Source: CAD feature listing. Evaluate the final solid. Frame: model axes, mm. Give positions to 0.01 mm unless a question says otherwise; leave off trailing zeros. Write each loop counter-clockwise with the first axis right and the second up, starting at its lowest first coordinate (ties: lowest second). Pieces come first, ordered by that corner, then holes. Notation, with made-up numbers: M 40.5,36.5 L 93.5,36.5 A38 ccw 93.5,75.5 Z; hole C 67.25,55.5 d6. An arc over 180 degrees is marked long. Use CSV: the item, a comma, the result in double quotes. Start each with the question number.
from build123d import *

# Parameters (mm, degrees)
F0_R     = 3.302961
F1_DEPTH = 3.81
F2_R     = 2.241818
F3_DEPTH = 12.7
F4_R     = 3.347199
F5_DEPTH = 3.81


with BuildPart() as f1:
    # F0 (on Front) → F1 (new body)
    with BuildSketch(Plane.XZ):
        Circle(F0_R)
    extrude(amount=-F1_DEPTH)

    # F2 (on face) → F3 (join)
    with BuildSketch(Plane(origin=(0, 3.81, 0), x_dir=(-1, 0, 0), z_dir=(0, 1, 0))):
        Circle(F2_R)
    extrude(amount=F3_DEPTH)

    # F4 (on face) → F5 (join)
    with BuildSketch(Plane(origin=(0, 16.51, 0), x_dir=(-1, 0, 0), z_dir=(0, 1, 0))):
        Circle(F4_R)
    extrude(amount=F5_DEPTH)


solid = f1.part
1. Section A-A on z = 3. Return loops of the section in (x, y), then the cut area to 3 significant figures.
2. First-contact query: pin 1 (4 mm diameter, centred on y = 13.5, z = 0.5, fed in from -X). Flat tip, straight axial feed; report the tip coordinate or a pass-through.
3. Section D-D on y = 13.75. Return loops of the section in (x, z), then the cut area to 3 significant figures.
4. Section B-B on x = 0. Return loops of the section in (y, z), then the cut area to 3 significant figures.
5. Section C-C on z = 0. Return loops of the section in (x, y), then the cut area to 3 significant figures.
6. Pull-direction query (Y, two-part tool) for faces 1 (the flat face through (0, 0, 0)), 2 (the flat face through (0, 20.32, 0)), 3 (the cylindrical face through (3.15, 1.88, 0.99)), 4 (the cylindrical face through (0.486, 10.071, -2.189)); classes: released by +Y, released by -Y, zero draft, split by the parting line, or undercut.
7. Line query: probe 1 along Y at (x, z) = (2, -2); probe 2 along X at (y, z) = (17.25, -0.75); probe 3 along Z at (x, y) = (-2.25, 3). Output: solid intervals per line, ascending.
Resolved:
1,outline,"M -1.48,16.51 L 1.48,16.51 L 1.48,20.32 L -1.48,20.32 Z; M -1.38,0 L 1.38,0 L 1.38,3.81 L -1.38,3.81 Z"
1,area,"21.8 mm2"
2,pin 1,"stops at x = -2.24"
3,outline,"C 0,0 d4.48"
3,area,"15.8 mm2"
4,outline,"M 0,-3.3 L 3.81,-3.3 L 3.81,-2.24 L 16.51,-2.24 L 16.51,-3.35 L 20.32,-3.35 L 20.32,3.35 L 16.51,3.35 L 16.51,2.24 L 3.81,2.24 L 3.81,3.3 L 0,3.3 Z"
4,area,"108 mm2"
5,outline,"M -3.35,16.51 L -2.24,16.51 L -2.24,3.81 L -3.3,3.81 L -3.3,0 L 3.3,0 L 3.3,3.81 L 2.24,3.81 L 2.24,16.51 L 3.35,16.51 L 3.35,20.32 L -3.35,20.32 Z"
5,area,"108 mm2"
6,face 1,"released by -Y"
6,face 2,"released by +Y"
6,face 3,"zero draft"
6,face 4,"undercut"
7,probe 1,"y = 0 to 3.81, 16.51 to 20.32"
7,probe 2,"x = -3.26 to 3.26"
7,probe 3,"z = -2.42 to 2.42"
